Read the model definition and answer for the solid it produces. Units are mm, in the model's axes. Face numbers are marked on the shaded views. A direction names the side the tool comes from. Coordinates: 2 decimals unless noted, no trailing zeros. Order: outer loops, then holes, each group sorted by start corner. A loop starts at its lowest first (then second) coordinate and runs counter-clockwise, first axis right, second up. Notation, with made-up numbers: (11.25, 9) -> (69.25, 9) arc R25 ccw to (69.25, 28) -> close; hole circle Ø1 at (-26, 79). An arc over 180 degrees is marked (long way). Answer in a Markdown table with one row per item.
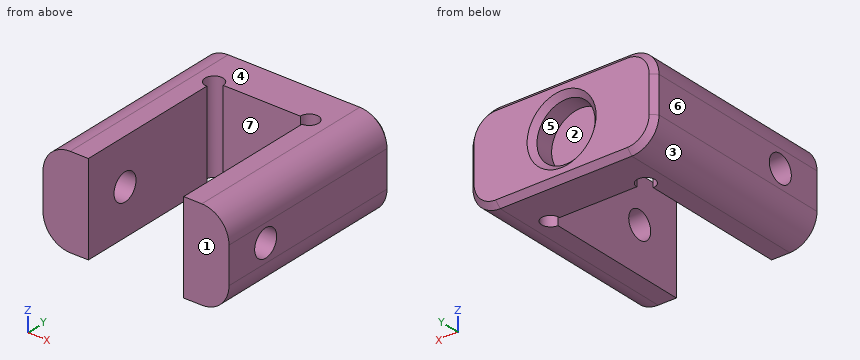
from build123d import *

# Parameters (mm, degrees)
EXTRUDE_1_DEPTH     = 10
SKETCH_2_R          = 3.2
CUT_EXTRUDE_1_DEPTH = 2.6
SKETCH_3_R          = 1.5
CUT_EXTRUDE_2_DEPTH = 26.355583705
FILLET_1_R          = 3
CHAMFER_1_SIZE      = 0.6
SKETCH_4_R          = 1
CUT_EXTRUDE_3_DEPTH = 19.102986632


with BuildPart() as part:
    # ｽｹｯﾁ1 → ﾎﾞｽ - 押し出し1 (new body)
    with BuildSketch(Plane.XY):
        Polygon((-10.25, 11.075), (-10.25, -11.075), (-5.25, -11.075), (-5.25, 6.075), (5.25, 6.075), (5.25, -11.075), (10.25, -11.075), (10.25, 11.075), align=None)
    extrude(amount=EXTRUDE_1_DEPTH)

    # ｽｹｯﾁ2 → ｶｯﾄ - 押し出し1 (cut)
    with BuildSketch(Plane(origin=(0, 11.075, 0), x_dir=(1, 0, 0), z_dir=(0, 1, 0))):
        with Locations(Location((0, -5, 0), (0, 0, 180))):
            Circle(SKETCH_2_R)
    extrude(amount=-CUT_EXTRUDE_1_DEPTH, mode=Mode.SUBTRACT)

    # ｽｹｯﾁ3 → ｶｯﾄ - 押し出し2 (cut, through all)
    with BuildSketch(Plane(origin=(10.25, 0, 0), x_dir=(0, 0, -1), z_dir=(1, 0, 0))):
        with Locations(Location((-5, -6.075, 0), (0, 0, 90))):
            Circle(SKETCH_3_R)
    extrude(amount=-CUT_EXTRUDE_2_DEPTH, mode=Mode.SUBTRACT)

    # ﾌｨﾚｯﾄ1
    fillet_1_edges = [part.edges().sort_by_distance(p)[0] for p in [
        (-10.25, 0, 0),
        (10.25, 0, 0),
        (10.25, 0, 10),
        (-10.25, 0, 10),
    ]]
    fillet(fillet_1_edges, radius=FILLET_1_R)

    # 面取り1
    chamfer_1_edges = [part.edges().sort_by_distance(p)[0] for p in [
        (3.2, 11.075, 5),
        (-10.25, 11.075, 5),
        (0, 11.075, 0),
        (0, 11.075, 10),
        (10.25, 11.075, 5),
        (9.371320344, 11.075, 9.121320344),
        (9.371320344, 11.075, 0.878679656),
        (-9.371320344, 11.075, 0.878679656),
        (-9.371320344, 11.075, 9.121320344),
    ]]
    chamfer(chamfer_1_edges, length=CHAMFER_1_SIZE)

    # ｽｹｯﾁ4 → ｶｯﾄ - 押し出し3 (cut, through all)
    with BuildSketch(Plane.XY.offset(10)):
        with Locations((5.25, 6.075)):
            Circle(SKETCH_4_R)
        with Locations((-5.25, 6.075)):
            Circle(SKETCH_4_R)
    extrude(amount=-CUT_EXTRUDE_3_DEPTH, mode=Mode.SUBTRACT)


solid = part.part
Q1. The part is cut by section C-C (x = 0). Write down the section's boundary in (y, z) (3 decimals).
Outcome:
| item | result |
|---|---|
| outline | (6.075, 0) -> (10.475, 0) -> (11.075, 0.6) -> (11.075, 1.2) -> (10.475, 1.8) -> (8.475, 1.8) -> (8.475, 8.2) -> (10.475, 8.2) -> (11.075, 8.8) -> (11.075, 9.4) -> (10.475, 10) -> (6.075, 10) -> close |
Q2. The part is cut by section A-A (y = 1.5). Write down the section's boundary in (x, z).
Outcome:
| item | result |
|---|---|
| outline | (-10.25, 3) arc R3 ccw to (-7.25, 0) -> (-5.25, 0) -> (-5.25, 10) -> (-7.25, 10) arc R3 ccw to (-10.25, 7) -> close; (5.25, 0) -> (7.25, 0) arc R3 ccw to (10.25, 3) -> (10.25, 7) arc R3 ccw to (7.25, 10) -> (5.25, 10) -> close |
Q3. Given pin 1 (4 mm diameter, centred on x = -1, z = 5.5, fed in from -Y) (3 decimals); pin 2 (4 mm diameter, centred on x = 0, z = 5, fed in from +Y) (3 decimals); pin 3 (5 mm diameter, centred on x = 0, z = 6, fed in from +Y) (3 decimals), each flat-ended and moving along its own axis, determine where each tip first touches the part or whether it passes through.
Outcome:
| item | result |
|---|---|
| pin 1 | y = 6.075 |
| pin 2 | y = 8.475 |
| pin 3 | y = 10.775 |
Q4. For the marked faces 5, 6 and 7, determine the directions among +Z, -Z, +X, -X, +Y, -Y from which every point of the face is accessible in a straight line to the end or side of a thin tool.
Outcome:
| item | result |
|---|---|
| face 5 | +Y |
| face 6 | +Z, -Z, -X, +Y, -Y |
| face 7 | +Z, -Z, -Y |
Q5. The part is cut by section B-B (z = 5). Write down the section's boundary in (x, y) (3 decimals).
Outcome:
| item | result |
|---|---|
| outline | (-10.25, -11.075) -> (-5.25, -11.075) -> (-5.25, -7.575) -> (-10.25, -7.575) -> close; (-10.25, -4.575) -> (-5.25, -4.575) -> (-5.25, 5.075) arc R1 cw (long way) to (-4.25, 6.075) -> (4.25, 6.075) arc R1 cw (long way) to (5.25, 5.075) -> (5.25, -4.575) -> (10.25, -4.575) -> (10.25, 10.475) -> (9.65, 11.075) -> (3.8, 11.075) -> (3.2, 10.475) -> (3.2, 8.475) -> (-3.2, 8.475) -> (-3.2, 10.475) -> (-3.8, 11.075) -> (-9.65, 11.075) -> (-10.25, 10.475) -> close; (5.25, -11.075) -> (10.25, -11.075) -> (10.25, -7.575) -> (5.25, -7.575) -> close |
Q6. Consider line 1 (Z direction, x = 0, y = 9.6); line 2 (X direction, y = 5, z = 3.5). Determine where each line is inside the solid, lowest interval first.
Outcome:
| item | result |
|---|---|
| line 1 | 0 to 1.8, 8.2 to 10 |
| line 2 | -10.25 to -5.25, 5.25 to 10.25 |
Q7. For a pull along Z with two mould halves and no side action, classify the marked faces 1, 2, 3 and 4 as pulls with the +Z half, pulls with the -Z half, needs draft (parallel to the pull), parting line crosses it, or undercut.
Outcome:
| item | result |
|---|---|
| face 1 | needs draft |
| face 2 | undercut |
| face 3 | pulls with the -Z half |
| face 4 | pulls with the +Z half |
